```python
from build123d import *

# Parameters (mm, degrees)
BOSS_EXTRUDE1_DEPTH             = 11.1125
F_1_4_CLEARANCE_HOLE1_D         = 6.7564
FILLET1_R                       = 1.5875
TAP_DRILL_FOR_1_4_20_TAP1_D     = 5.1054
TAP_DRILL_FOR_1_4_20_TAP1_DEPTH = 9.525
TAP_DRILL_FOR_1_4_20_TAP1_TIP   = 1.533816902


with BuildPart() as part:
    # Sketch1 → Boss-Extrude1 (new, symmetric)
    with BuildSketch(Plane.XY):
        Polygon((0, 0), (25.4, 0), (25.4, 6.35), (0, 6.35), (0, 13.269040681), (-37.087633685, -12.7), (-3.175, -12.7), (-3.175, 0), align=None)
    extrude(amount=BOSS_EXTRUDE1_DEPTH, both=True)

    # 1/4 Clearance Hole1 (through all)
    with Locations(Plane(origin=(0, 6.35, 0), x_dir=(1, 0, 0), z_dir=(0, 1, 0))):
        with Locations((6.35, 4.7625), (20.6375, 4.7625), (6.35, -4.7625), (20.6375, -4.7625)):
            Hole(F_1_4_CLEARANCE_HOLE1_D / 2)

    # Fillet1
    fillet1_edges = [part.edges().sort_by_distance(p)[0] for p in [
        (-3.175, 0, 0),
        (-3.175, -12.7, 0),
        (-37.087633685, -12.7, 0),
        (0, 13.269040681, 0),
        (0, 6.35, 0),
    ]]
    fillet(fillet1_edges, radius=FILLET1_R)

    # Tap Drill for 1/4-20 Tap1
    with Locations(Plane(origin=(-6.234409806, 8.903659938, 0), x_dir=(0.8191520442889947, 0.5735764363510422, 0), z_dir=(-0.573576436351042, 0.8191520442889946, 0))):
        with Locations((-16.201690933, 6.35), (-3.501690933, 6.35), (-3.501690933, -6.35), (-16.201690933, -6.35)):
            Hole(TAP_DRILL_FOR_1_4_20_TAP1_D / 2, depth=TAP_DRILL_FOR_1_4_20_TAP1_DEPTH)
            with Locations((0, 0, -(TAP_DRILL_FOR_1_4_20_TAP1_DEPTH + TAP_DRILL_FOR_1_4_20_TAP1_TIP / 2))):  # 118° drill point
                Cone(0, TAP_DRILL_FOR_1_4_20_TAP1_D / 2, TAP_DRILL_FOR_1_4_20_TAP1_TIP, mode=Mode.SUBTRACT)


solid = part.part
```
Design review of the part built by this model. Coordinates are the model's own, in mm. A direction names the side the tool comes from. Give positions to 0.01 mm unless a question says otherwise; leave off trailing zeros. Write each loop counter-clockwise with the first axis right and the second up, starting at its lowest first coordinate (ties: lowest second). Pieces come first, ordered by that corner, then holes.
(1) Tool access review of faces 3 (the face through (-3.615, -2.223, -6.382)), 4 (the face through (12, 0, 0)), 5 (the face through (0, 9, 0)): name each direction out of +Z, -Z, +X, -X, +Y, -Y from which nothing blocks a thin tool from reaching the whole face with its end or side.
Checked values:
face 3: none
face 4: +Z, -Z, +X, -Y
face 5: +Z, -Z, +X, +Y
(2) Add section A-A (x = 6.35). Give the boundary of the cut face in (y, z), and give its area (3 significant figures).
Checked values:
outline: (0, -11.11) - (6.35, -11.11) - (6.35, -8.14) - (0, -8.14) - close; (0, -1.38) - (6.35, -1.38) - (6.35, 1.38) - (0, 1.38) - close; (0, 8.14) - (6.35, 8.14) - (6.35, 11.11) - (0, 11.11) - close
area: 55.3 mm2
(3) Clearance check with flat-ended pins moving along their axes: pin 1 Ø1 at (x, z) = (11, -5.5) entering from +Y; pin 2 Ø12 at (x, z) = (12, -9) entering from -Y; pin 3 Ø2 at (y, z) = (-1.5, -4) entering from -X. State where each tip first meets the part, or that it passes through.
Checked values:
pin 1: stops at y = 6.35
pin 2: stops at y = 0
pin 3: stops at x = -22.52
(4) Wall thickness on line 1 along Z through (x, y) = (6.35, 1.75); line 2 along X through (y, z) = (3, 2.25); line 3 along X through (y, z) = (6, 7): over which ranges is each line inside the solid? List them lowest first.
Checked values:
line 1: z = -11.11 to -8.14, -1.38 to 1.38, 8.14 to 11.11
line 2: x = -14.67 to 4.09, 8.61 to 18.38, 22.9 to 25.4
line 3: x = -5.46 to 3.82, 8.88 to 18.11, 23.17 to 25.4
(5) Add section C-C (z = -3.25). Give the number of separate pieces and of enclosed holes in the cut face, and give its area (3 significant figures).
Checked values:
separate pieces: 3
enclosed holes: 0
area: 519 mm2
(6) Add section D-D (y = 9.25). Give the boundary of the cut face in (x, z), and give its area (3 significant figures).
Checked values:
outline: (-5.74, -11.11) - (0, -11.11) - (0, 11.11) - (-5.74, 11.11) - close
area: 128 mm2
(7) Mouldability with a two-part tool opening along Z and no side actions: class faces 1 (the face through (-19, -12.7, 0)), 2 (the face through (17.52, 3.13, 6.06)) as +Z half, -Z half, draft (parallel to the pull), parting line (faces both ways), or undercut.
Checked values:
face 1: draft
face 2: undercut
